For this review, take the finished solid that the model builds, in its own axes (mm). Coordinates: 2 decimals unless noted, no trailing zeros. Loops run counter-clockwise (first coordinate to the right, second up) from the corner with the lowest first, then second, coordinate; pieces in that order, holes last. Notation, with made-up numbers: M -19,27.5 L -15,27.5 A31 cw -15,51.5 Z; hole C 12.5,-0.5 d9. An arc over 180 degrees is marked long. Write item = value, one per line.
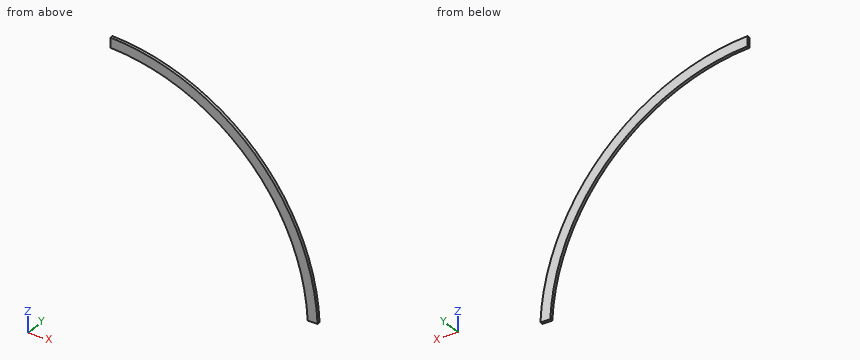
from build123d import *

# Parameters (mm, degrees)
SKETCH1_R            = 220
SKETCH1_R_2          = 210
BOSS_EXTRUDE1_DEPTH  = 1.5
QUADRUPLE_DEPTH      = 312.130599588
QUADRUPLE_DEPTH_BACK = 312.130599588
SKETCH2_W            = 20
SKETCH2_H            = 440
SKETCH2_W_2          = 440
SKETCH2_H_2          = 20
SKETCH4_W            = 439.545219516
SKETCH4_H            = 3
HALF_DEPTH           = 311.809024965
SKETCH5_W            = 439.545219516
SKETCH5_H            = 3
QUARTER_DEPTH        = 311.809024965


with BuildPart() as part:
    # Sketch1 → Boss-Extrude1 (new, symmetric)
    with BuildSketch(Plane(origin=(0, 0, 0), x_dir=(1, 0, 0), z_dir=(0, 1, 0))):
        with Locations(Location((0, 0, 0), (0, 0, 270))):
            Circle(SKETCH1_R)
        with Locations(Location((0, 0, 0), (0, 0, 270))):
            Circle(SKETCH1_R_2, mode=Mode.SUBTRACT)
    extrude(amount=BOSS_EXTRUDE1_DEPTH, both=True)

    # Sketch2 → quadruple (cut, two sides: drawn at the far end of the back side and taken through both)
    with BuildSketch(Plane(origin=(0, 0, 0), x_dir=(1, 0, 0), z_dir=(0, 1, 0)).offset(-QUADRUPLE_DEPTH_BACK)):
        Rectangle(SKETCH2_W, SKETCH2_H)
        Rectangle(SKETCH2_W_2, SKETCH2_H_2)
    extrude(amount=QUADRUPLE_DEPTH + QUADRUPLE_DEPTH_BACK, mode=Mode.SUBTRACT)


with BuildPart() as quadruple_piece_1:
    # of the separate pieces the step leaves, piece 1, a body of its own (quadruple_pieces)
    add(part.part.solids().sort_by_distance((-219.772609758, -1.5, 10))[0])

    # Sketch5 → quarter (cut, through all)
    with BuildSketch(Plane(origin=(0, 0, 0), x_dir=(0, 0, -1), z_dir=(1, 0, 0))):
        Rectangle(SKETCH5_W, SKETCH5_H)
    extrude(amount=-QUARTER_DEPTH, mode=Mode.SUBTRACT)


with BuildPart() as quadruple_piece_2:
    # of the separate pieces the step leaves, piece 2, a body of its own (quadruple_pieces)
    add(part.part.solids().sort_by_distance((-10, 1.5, -219.772609758))[0])


with BuildPart() as quadruple_piece_3:
    # of the separate pieces the step leaves, piece 3, a body of its own (quadruple_pieces)
    add(part.part.solids().sort_by_distance((10, -1.5, 219.772609758))[0])


with BuildPart() as quadruple_piece_4:
    # of the separate pieces the step leaves, piece 4, a body of its own (quadruple_pieces)
    add(part.part.solids().sort_by_distance((209.761769634, 1.5, -10))[0])


with BuildPart() as half_tool:
    # Sketch4 → half (new, through all)
    with BuildSketch(Plane.XY):
        Rectangle(SKETCH4_W, SKETCH4_H)
    extrude(amount=-HALF_DEPTH)


with BuildPart() as quadruple_piece_2_1:
    add(quadruple_piece_2.part)

    # half: cut by half_tool
    add(half_tool.part, mode=Mode.SUBTRACT)


with BuildPart() as quadruple_piece_4_1:
    add(quadruple_piece_4.part)

    # half: cut by half_tool
    add(half_tool.part, mode=Mode.SUBTRACT)


solid = quadruple_piece_3.part
Q1. For line 1 along Z through (x, y) = (122, 0.6); line 2 along Z through (x, y) = (125, -1.05); line 3 along X through (y, z) = (1.3, 159), list the stretches that pass through material, from the lowest coordinate up.
Solved:
line_1 = 170.93 to 183.07
line_2 = 168.75 to 181.04
line_3 = 137.18 to 152.05
Q2. Add section A-A (y = -0.8). Write out the cut boundary in (x, z), and give its area (3 significant figures).
Solved:
outline = M 10,209.76 A210 cw 209.76,10 L 219.77,10 A220 ccw 10,219.77 Z
area = 3,180 mm²
Q3. Add section B-B (z = 134). Write out the cut boundary in (x, y), and give its area (3 significant figures).
Solved:
outline = M 161.69,-1.5 L 174.48,-1.5 L 174.48,1.5 L 161.69,1.5 Z
area = 38.4 mm²
Q4. For pin 1 Ø1.5 at (x, y) = (119, -1) entering from -Z; pin 2 Ø1 at (x, y) = (94, -0.5) entering from +Z, all flat-tipped, find the tip position at first contact; note any pin that passes through.
Solved:
pin_1 = 172.51
pin_2 = 199.14
